Design review of the part shown in the three views and the two pictorial views. Dimensions are in mm from the part's minimum x, y and z. A direction names the side the tool comes from. Round coordinates to 2 decimals unless told otherwise and drop trailing zeros. Loops run counter-clockwise (first coordinate to the right, second up) from the corner with the lowest first, then second, coordinate; pieces in that order, holes last. Notation, with made-up numbers: M -21.75,61 L 16.25,61 A27 ccw 16.25,91 Z; hole C 87,-21.5 d9. An arc over 180 degrees is marked long. One line per question, with ' | ' between items.
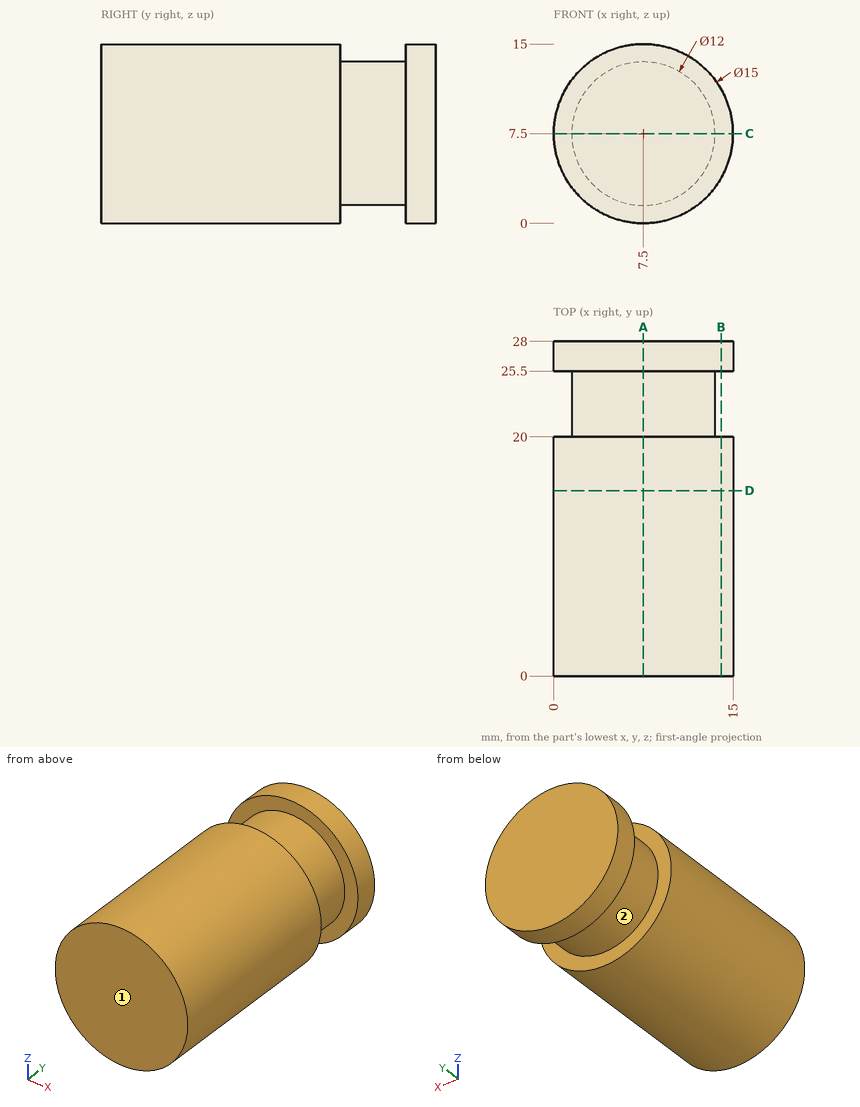
1) Add section B-B on x = 14. State the section outline as (y, z) points.
Output values:
outline: M 0,3.76 L 20,3.76 L 20,11.24 L 0,11.24 Z; M 25.5,3.76 L 28,3.76 L 28,11.24 L 25.5,11.24 Z
2) Add section C-C on z = 7.5. State the section outline as (x, y) points.
Output values:
outline: M 0,0 L 15,0 L 15,20 L 13.5,20 L 13.5,25.5 L 15,25.5 L 15,28 L 0,28 L 0,25.5 L 1.5,25.5 L 1.5,20 L 0,20 Z
3) Insertion check: P1, Ø1.5, axis at y = 10.5, z = 11.5, coming from the -X side; P2, Ø3, axis at y = 19.5, z = 5, coming from the -X side; P3, Ø1.5, axis at x = 3, y = 21, coming from the +Z side. Each pin has a flat end and moves straight along its axis. Give the tip position at first contact, or say it passes through.
Output values:
P1: stops at x = 0.74 | P2: stops at x = 0.07 | P3: stops at z = 12.18
4) Machinability: for the marked faces 1 and 2, which of the approach directions +Z, -Z, +X, -X, +Y, -Y give a long, thin tool a straight path to every point of the face, cutting with its end or side? Answer none if there is none.
Output values:
face 1: +Z, -Z, +X, -X, -Y | face 2: none
5) Add section A-A on x = 7.5. State the section outline as (y, z) points.
Output values:
outline: M 0,0 L 20,0 L 20,1.5 L 25.5,1.5 L 25.5,0 L 28,0 L 28,15 L 25.5,15 L 25.5,13.5 L 20,13.5 L 20,15 L 0,15 Z
6) Add section D-D on y = 15.5. State the section outline as (x, z) points, then the cut area to 3 significant figures.
Output values:
outline: C 7.5,7.5 d15 | area: 177 mm²
7) For line 1 (Y direction, x = 13.5, z = 6.5); line 2 (X direction, y = 7.75, z = 7.75); line 3 (Z direction, x = 5, y = 24.25), list the stretches that pass through material, from the lowest coordinate up.
Output values:
line 1: y = 0 to 20, 25.5 to 28 | line 2: x = 0 to 15 | line 3: z = 2.05 to 12.95
